For this review, take the finished solid that the model builds, in its own axes (mm). A direction names the side the tool comes from. Round coordinates to 2 decimals unless told otherwise and drop trailing zeros. Order: outer loops, then holes, each group sorted by start corner. A loop starts at its lowest first (then second) coordinate and runs counter-clockwise, first axis right, second up. Notation, with made-up numbers: (45, 33) - (82, 33) arc R34 cw to (82, 67) - close; hole circle Ø11 at (-25, -26). An arc over 180 degrees is marked (long way). One line per item, written item: value.
Autodesk Inventor part; units mm, degrees
ref_plane "YZ Plane" through (0, 0, 0) normal (1, 0, 0) x (0, 1, 0)
ref_plane "XZ Plane" through (0, 0, 0) normal (0, 1, 0) x (-1, 0, 0)
ref_plane "XY Plane" through (0, 0, 0) normal (0, 0, 1) x (1, 0, 0)
sketch "スケッチ1" plane through (0, 0, 0) normal (0, 0, 1) x (1, 0, 0)
  line L0 (0, 0) -> (-65, 0)
  line L1 (-65, 0) -> (-65, -60)
  line L2 (-65, -60) -> (0, -60)
  line L3 (0, -60) -> (0, 0)
  dimension "d0" = 65
  dimension "d1" = 60
extrude "押し出し1" add sketch "スケッチ1" along normal blind 3
sketch "スケッチ2" plane through (0, 0, 3) normal (0, 0, 1) x (1, 0, 0)
  line L0 (-29, -25.6891) -> (-49.829, 0)
  line L1 (-2.171, 0) -> (-23, -25.6891)
  line L2 (-62, -31) -> (-65, -31)
  line L3 (-65, -31) -> (-65, -25)
  line L4 (-65, -25) -> (-62, -25)
  line L5 (-62, -25) -> (-62, -31)
  line L6 (-62, -17) -> (-65, -17)
  line L7 (-65, -17) -> (-65, -11)
  line L8 (-65, -11) -> (-62, -11)
  line L9 (-62, -11) -> (-62, -17)
  line L10 (-65, 4) -> (-62, 4)
  line L11 (-62, 4) -> (-62, 0)
  line L12 (-62, 0) -> (-65, 0)
  line L13 (-65, -4) -> (-65, 0)
  line L14 (-62, -4) -> (-65, -4)
  line L15 (-62, 0) -> (-62, -4)
  line L16 (-65, 0) -> (-65, 4)
  line L17 (-65, -40) -> (-62, -40)
  line L18 (0, 0) -> (0, -60)
  line L19 (0, -60) -> (-65, -60)
  line L20 (-65, -60) -> (-65, 0)
  line L21 (-65, 0) -> (0, 0)
  line L22 (-49.829, 0) -> (-62, -11)
  arc A0 (-29, -32.3891) -> (-23, -32.3891) centre (-26, -32.3891) ccw
  line L23 (-26, -32.3891) -> (-26, -29.3891) construction
  circle A1 centre (-26, -32.3891) radius 1.25
  line L24 (-23, -32.3891) -> (-23, -25.6891)
  line L25 (-29, -32.3891) -> (-29, -25.6891)
  circle A2 centre (-26, -18.3891) radius 1.25
  circle A3 centre (-26, -6.3891) radius 1.25
  line L26 (-29, -25.6891) -> (-62, -31)
  dimension "d4" = 6
  dimension "d5" = 2.5
  dimension "d6" = 3
  dimension "d7" = 2.5
  dimension "d8" = 2.5
  dimension "d9" = 14
  dimension "d10" = 26
extrude "押し出し2" cut sketch "スケッチ2" against normal blind 3 contours L26 L5 L4 L20 L6 L9 L22 L0 | L0 L21 L1 L24 A0 L25 keep common part
sketch "スケッチ3" plane through (0, 0, 3) normal (0, 0, 1) x (1, 0, 0)
  circle A0 centre (-26, -6.3891) radius 1.25
  circle A1 centre (-26, -18.3891) radius 1.25
  circle A2 centre (-26, -32.3891) radius 1.25
  line L0 (-62, -25) -> (-65, -25)
  line L1 (-65, -25) -> (-65, -17)
  line L2 (-65, -17) -> (-62, -17)
  line L3 (-62, -17) -> (-62, -11)
  line L4 (-62, -11) -> (-49.829, 0)
  line L5 (-49.829, 0) -> (-2.171, 0)
  line L6 (-2.171, 0) -> (-23, -25.6891)
  line L7 (-23, -25.6891) -> (-23, -32.3891)
  arc A3 (-29, -32.3891) -> (-23, -32.3891) centre (-26, -32.3891) ccw
  line L8 (-29, -32.3891) -> (-29, -25.6891)
  line L9 (-29, -25.6891) -> (-62, -31)
  line L10 (-62, -31) -> (-62, -25)
  arc A4 (-62, -28.9881) -> (-62, -27.7881) centre (-62.8, -28.3881) ccw
  arc A5 (-62, -14.6) -> (-62, -13.4) centre (-62.8, -14) ccw
  point P0 (0, 0)
  dimension "d13" = 2
  dimension "d14" = 2
  dimension "d15" = 3
  dimension "d16" = 3.3881
  dimension "d17" = 0.8
extrude "押し出し3" cut sketch "スケッチ3" against normal blind 3 contours A4 L10 | L3 A5
sketch "スケッチ4" plane through (0, 0, 3) normal (0, 0, 1) x (1, 0, 0)
  circle A0 centre (-26, -6.3891) radius 1.25
  circle A1 centre (-26, -18.3891) radius 1.25
  circle A2 centre (-26, -32.3891) radius 1.25
  line L0 (-29, -32.3891) -> (-29, -25.6891)
  line L1 (-29, -25.6891) -> (-62, -31)
  line L2 (-62, -31) -> (-62, -28.9881)
  arc A3 (-62, -28.9881) -> (-62, -27.7881) centre (-62.8, -28.3881) ccw
  line L3 (-62, -27.7881) -> (-62, -25)
  line L4 (-62, -25) -> (-65, -25)
  line L5 (-65, -25) -> (-65, -17)
  line L6 (-65, -17) -> (-62, -17)
  line L7 (-62, -17) -> (-62, -14.6)
  arc A4 (-62, -14.6) -> (-62, -13.4) centre (-62.8, -14) ccw
  line L8 (-62, -13.4) -> (-62, -11)
  line L9 (-62, -11) -> (-49.829, 0)
  line L10 (-49.829, 0) -> (-2.171, 0)
  line L11 (-2.171, 0) -> (-23, -25.6891)
  line L12 (-23, -25.6891) -> (-23, -32.3891)
  arc A5 (-29, -32.3891) -> (-23, -32.3891) centre (-26, -32.3891) ccw
  line L13 (-58, -25) -> (-61, -25)
  line L14 (-61, -25) -> (-61, -17)
  line L15 (-61, -17) -> (-58, -17)
  line L16 (-65, -17) -> (-65, -25)
  line L17 (-62, -25) -> (-65, -25)
  circle A6 centre (-58.8, -28.3881) radius 1
  circle A7 centre (-58.8, -14) radius 1
  arc A8 (-62, -14.6) -> (-62, -13.4) centre (-62.8, -14) ccw
  line L18 (-49.829, 0) -> (-58, -11)
  line L19 (-58, -31) -> (-29, -25.6891)
  line L20 (-29, -25.6891) -> (-49.829, 0)
  line L21 (-58, -31) -> (-58, -28.9881)
  line L22 (-58, -27.7881) -> (-58, -25)
  line L23 (-58, -17) -> (-58, -14.6)
  line L24 (-58, -13.4) -> (-58, -11)
  dimension "d26" = 3
  dimension "d27" = 6
  dimension "d28" = 6
  dimension "d29" = 4
sketch "スケッチ5" plane through (0, 0, 3) normal (0, 0, 1) x (1, 0, 0)
  circle A0 centre (-26, -6.3891) radius 1.25
  circle A1 centre (-26, -18.3891) radius 1.25
  circle A2 centre (-26, -32.3891) radius 1.25
  line L0 (-29, -32.3891) -> (-29, -25.6891)
  line L1 (-29, -25.6891) -> (-62, -31)
  line L2 (-62, -31) -> (-62, -28.9881)
  arc A3 (-62, -28.9881) -> (-62, -27.7881) centre (-62.8, -28.3881) ccw
  line L3 (-62, -27.7881) -> (-62, -25)
  line L4 (-62, -25) -> (-65, -25)
  line L5 (-65, -25) -> (-65, -17)
  line L6 (-65, -17) -> (-62, -17)
  line L7 (-62, -17) -> (-62, -14.6)
  arc A4 (-62, -14.6) -> (-62, -13.4) centre (-62.8, -14) ccw
  line L8 (-62, -13.4) -> (-62, -11)
  line L9 (-62, -11) -> (-49.829, 0)
  line L10 (-49.829, 0) -> (-2.171, 0)
  line L11 (-2.171, 0) -> (-23, -25.6891)
  line L12 (-23, -25.6891) -> (-23, -32.3891)
  arc A5 (-29, -32.3891) -> (-23, -32.3891) centre (-26, -32.3891) ccw
  circle A6 centre (-26, -6.3891) radius 1.25
  circle A7 centre (-26, -18.3891) radius 1.25
  circle A8 centre (-26, -32.3891) radius 1.25
  line L13 (-29, -32.3891) -> (-29, -25.6891)
  line L14 (-29, -25.6891) -> (-62, -31)
  line L15 (-62, -31) -> (-62, -28.9881)
  arc A9 (-62, -28.9881) -> (-62, -27.7881) centre (-62.8, -28.3881) ccw
  line L16 (-62, -27.7881) -> (-62, -25)
  line L17 (-62, -25) -> (-65, -25)
  line L18 (-65, -25) -> (-65, -17)
  line L19 (-65, -17) -> (-62, -17)
  line L20 (-62, -17) -> (-62, -14.6)
  arc A10 (-62, -14.6) -> (-62, -13.4) centre (-62.8, -14) ccw
  line L21 (-62, -13.4) -> (-62, -11)
  line L22 (-62, -11) -> (-49.829, 0)
  line L23 (-49.829, 0) -> (-2.171, 0)
  line L24 (-2.171, 0) -> (-23, -25.6891)
  line L25 (-23, -25.6891) -> (-23, -32.3891)
  arc A11 (-29, -32.3891) -> (-23, -32.3891) centre (-26, -32.3891) ccw
  circle A12 centre (-26, -6.3891) radius 1.25
  circle A13 centre (-26, -18.3891) radius 1.25
  circle A14 centre (-26, -32.3891) radius 1.25
  line L26 (-29, -32.3891) -> (-29, -25.6891)
  line L27 (-29, -25.6891) -> (-62, -31)
  line L28 (-62, -31) -> (-62, -28.9881)
  arc A15 (-62, -28.9881) -> (-62, -27.7881) centre (-62.8, -28.3881) ccw
  line L29 (-62, -27.7881) -> (-62, -25)
  line L30 (-62, -25) -> (-65, -25)
  line L31 (-65, -25) -> (-65, -17)
  line L32 (-65, -17) -> (-62, -17)
  line L33 (-62, -17) -> (-62, -14.6)
  arc A16 (-62, -14.6) -> (-62, -13.4) centre (-62.8, -14) ccw
  line L34 (-62, -13.4) -> (-62, -11)
  line L35 (-62, -11) -> (-49.829, 0)
  line L36 (-49.829, 0) -> (-2.171, 0)
  line L37 (-2.171, 0) -> (-23, -25.6891)
  line L38 (-23, -25.6891) -> (-23, -32.3891)
  arc A17 (-29, -32.3891) -> (-23, -32.3891) centre (-26, -32.3891) ccw
  arc A18 (-62, -14.6) -> (-62, -13.4) centre (-62.8, -14) ccw
  line L39 (-62, -17) -> (-62, -14.6)
  line L40 (-65, -17) -> (-62, -17)
  line L41 (-65, -17) -> (-65, -25)
  line L42 (-62, -25) -> (-65, -25)
  line L43 (-62, -27.7881) -> (-62, -25)
  arc A19 (-62, -28.9881) -> (-62, -27.7881) centre (-62.8, -28.3881) ccw
  line L44 (-62, -31) -> (-62, -28.9881)
  line L45 (-29, -25.6891) -> (-62, -31)
  line L46 (-29, -32.3891) -> (-29, -25.6891)
  arc A20 (-29, -32.3891) -> (-23, -32.3891) centre (-26, -32.3891) ccw
  line L47 (-23, -25.6891) -> (-23, -32.3891)
  line L48 (-2.171, 0) -> (-23, -25.6891)
  line L49 (-2.171, 0) -> (-49.829, 0)
  line L50 (-62, -11) -> (-49.829, 0)
  line L51 (-62, -13.4) -> (-62, -11)
  circle A21 centre (-26, -32.3891) radius 1.25
  circle A22 centre (-26, -18.3891) radius 1.25
  circle A23 centre (-26, -6.3891) radius 1.25
  line L52 (-29, -25.6891) -> (-49.829, 0)
  line L53 (-29, -25.6891) -> (-65.9346, -36.6422)
  line L54 (-65.9346, -36.6422) -> (-73.9425, -10.887)
  line L55 (-73.9425, -10.887) -> (-49.829, 0)
  point P0 (0, 0)
extrude "押し出し4" cut sketch "スケッチ5" against normal blind 3 contours L1 L2 A3 L3 L4 L5 L6 L7 A4 L8 L9 L52
extrude "押し出し5" add sketch "スケッチ4" against normal blind 3 contours L19 L21 L1 | L1 L21 A6 L22 L13 L14 L15 L23 A7 L24 L18 L20
equation "\"d28\" = d27"
properties part number "handPlate2"
Item 1: Machinability: for faces 1 (the flat face through (-23, -29, 2)), 2 (the flat face through (-58, -26, 2)), 3 (the flat face through (-43.7, -28.38, 1.52)), 4 (the flat face through (-60, -17, 2)), which of the approach directions +Z, -Z, +X, -X, +Y, -Y give a long, thin tool a straight path to every point of the face, cutting with its end or side? Answer none if there is none.
Returned:
face 1: +Z, -Z, +X, -Y
face 2: +Z, -Z, -X, -Y
face 3: +Z, -Z, -Y
face 4: +Z, -Z, -X, +Y
Item 2: For P1, Ø1.5, axis at y = -29.5, z = 1.5, coming from the +X side; P2, Ø1.2, axis at y = -15.5, z = 1.5, coming from the -X side; P3, Ø2, axis at x = -26, y = -32.39, coming from the +Z side; P4, Ø1.5, axis at x = -46.5, z = 2, coming from the -Y side, all flat-tipped, find the tip position at first contact; note any pin that passes through.
Returned:
P1: x = -23
P2: x = -58
P3: through
P4: y = -29.03
Item 3: Take a section at D-D (x = -34.5). Write out the cut boundary in (y, z).
Returned:
outline: (-26.7, 0) - (0, 0) - (0, 3) - (-26.7, 3) - close
Item 4: Take a section at C-C (y = -23). Write out the cut boundary in (x, z), plus the area to 3 significant figures.
Returned:
outline: (-61, 0) - (-20.82, 0) - (-20.82, 3) - (-61, 3) - close
area: 121 mm^2
Item 5: Take a section at B-B (z = 1.95). Write out the cut boundary in (x, y).
Returned:
outline: (-61, -25) - (-58, -25) - (-58, -27.79) arc R1 cw to (-58, -28.99) - (-58, -31) - (-29, -25.69) - (-29, -32.39) arc R3 ccw to (-23, -32.39) - (-23, -25.69) - (-2.17, 0) - (-49.83, 0) - (-58, -11) - (-58, -13.4) arc R1 cw to (-58, -14.6) - (-58, -17) - (-61, -17) - close; hole circle Ø2.5 at (-26, -32.39); hole circle Ø2.5 at (-26, -18.39); hole circle Ø2.5 at (-26, -6.39)
Item 6: Wall thickness on line 1 (Y direction, x = -26, z = 1.15); line 2 (Y direction, x = -25.5, z = 2.65); line 3 (X direction, y = -19, z = 0.65): over which ranges is each line inside the solid? List them lowest first.
Returned:
line 1: -35.39 to -33.64, -31.14 to -19.64, -17.14 to -7.64, -5.14 to 0
line 2: -35.35 to -33.53, -31.24 to -19.53, -17.24 to -7.53, -5.24 to 0
line 3: -61 to -27.09, -24.91 to -17.58
Item 7: The part is to be moulded in two halves that separate along X. For faces 5 (the flat face through (-58, -16, 2)), 6 (the flat face through (-29, -29, 2)), 7 (the cylindrical face through (-26.07, -35.39, 1.52)), say which applies: +X half, -X half, draft (parallel to the pull), parting line (faces both ways), or undercut.
Returned:
face 5: -X half
face 6: undercut
face 7: parting line
Item 8: Take a section at A-A (x = -26). Write out the cut boundary in (y, z), plus the area to 3 significant figures.
Returned:
outline: (-35.39, 0) - (-33.64, 0) - (-33.64, 3) - (-35.39, 3) - close; (-31.14, 0) - (-19.64, 0) - (-19.64, 3) - (-31.14, 3) - close; (-17.14, 0) - (-7.64, 0) - (-7.64, 3) - (-17.14, 3) - close; (-5.14, 0) - (0, 0) - (0, 3) - (-5.14, 3) - close
area: 83.7 mm^2
